Geometry: see drawing. Coordinates: mm, zero at the bounding-box minimum. Coordinates: 2 decimals unless noted, no trailing zeros. Order: outer loops, then holes, each group sorted by start corner. A loop starts at its lowest first (then second) coordinate and runs counter-clockwise, first axis right, second up. Notation, with made-up numbers: (1, 16.5) - (45, 16.5) arc R25 ccw to (45, 36.5) - close; hole circle Ø1 at (71, -2.5). An arc over 180 degrees is marked (long way). Use a Markdown table: item, result. Add a question column.
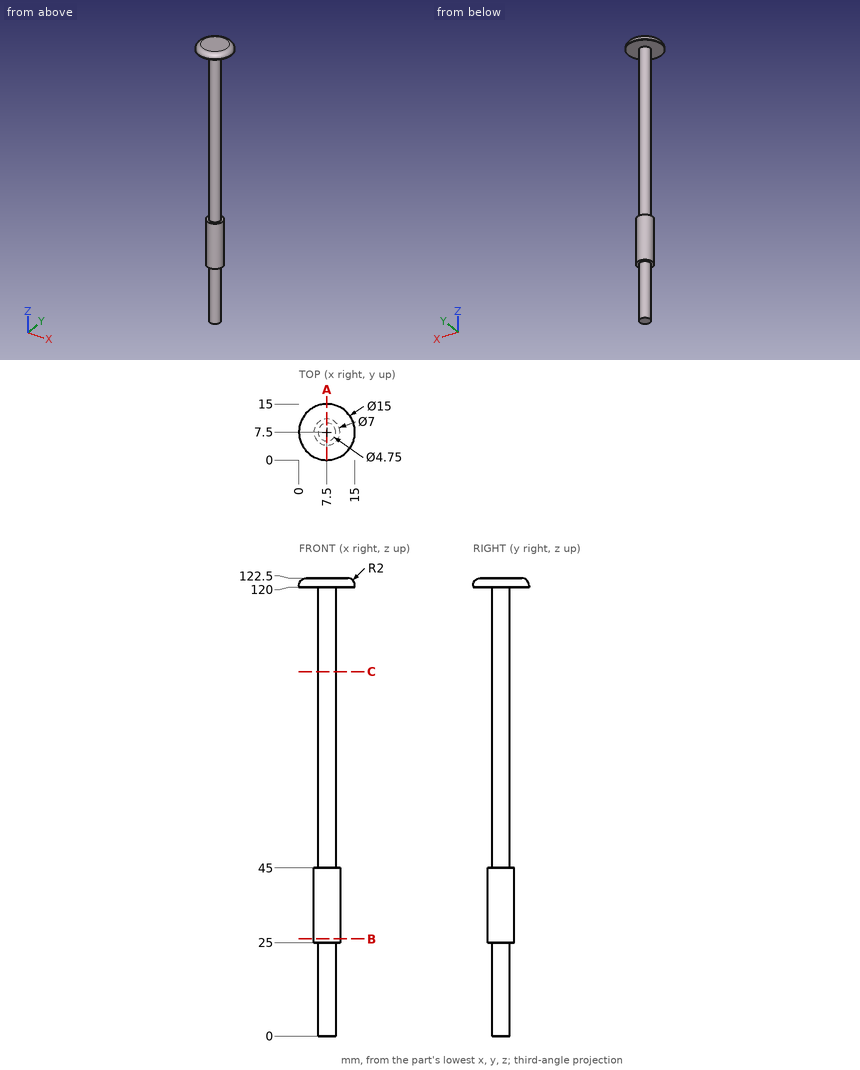
1) First-contact query: pin 1 (3 mm diameter, centred on y = 2.5, z = 75.5, fed in from -X); pin 2 (8 mm diameter, centred on y = 9.5, z = 54, fed in from -X) (3 decimals); pin 3 (6 mm diameter, centred on y = 4.5, z = 32, fed in from -X); pin 4 (6 mm diameter, centred on y = 3, z = 26.5, fed in from -X). Flat tips, straight axial feed; report the tip coordinate or a pass-through.
2) Section query B-B (z = 26). Return the cut outline in (x, y).
3) Line query: line 1 (Z direction, x = 8.25, y = 10); line 2 (Z direction, x = 6.25, y = 13); line 3 (Y direction, x = 7.25, z = 76.5). Output: solid intervals per line, ascending. Write a range as from..to.
4) Section query C-C (z = 97.5). Return the cut outline in (x, y) (3 decimals).
5) Section query A-A (x = 7.5). Return the cut outline in (y, z) (3 decimals).
From the geometry:
| question | item | result |
|---|---|---|
| 1 | pin 1 | passes through |
| 1 | pin 2 | stops at x = 5.125 |
| 1 | pin 3 | stops at x = 4 |
| 1 | pin 4 | stops at x = 4.34 |
| 2 | outline | circle Ø7 at (7.5, 7.5) |
| 3 | line 1 | z = 25..45, 120..122.5 |
| 3 | line 2 | z = 120..122.5 |
| 3 | line 3 | y = 5.14..9.86 |
| 4 | outline | circle Ø4.75 at (7.5, 7.5) |
| 5 | outline | (0, 120) - (5.125, 120) - (5.125, 45) - (4, 45) - (4, 25) - (5.125, 25) - (5.125, 0) - (9.875, 0) - (9.875, 25) - (11, 25) - (11, 45) - (9.875, 45) - (9.875, 120) - (15, 120) - (15, 120.5) arc R2 ccw to (13, 122.5) - (2, 122.5) arc R2 ccw to (0, 120.5) - close |
